Here's the drawing with two shaded views (mm, measured from the low corner). I have some questions. A direction names the side the tool comes from. Coordinates: 2 decimals unless noted, no trailing zeros. Write each loop counter-clockwise with the first axis right and the second up, starting at its lowest first coordinate (ties: lowest second). Pieces come first, ordered by that corner, then holes.
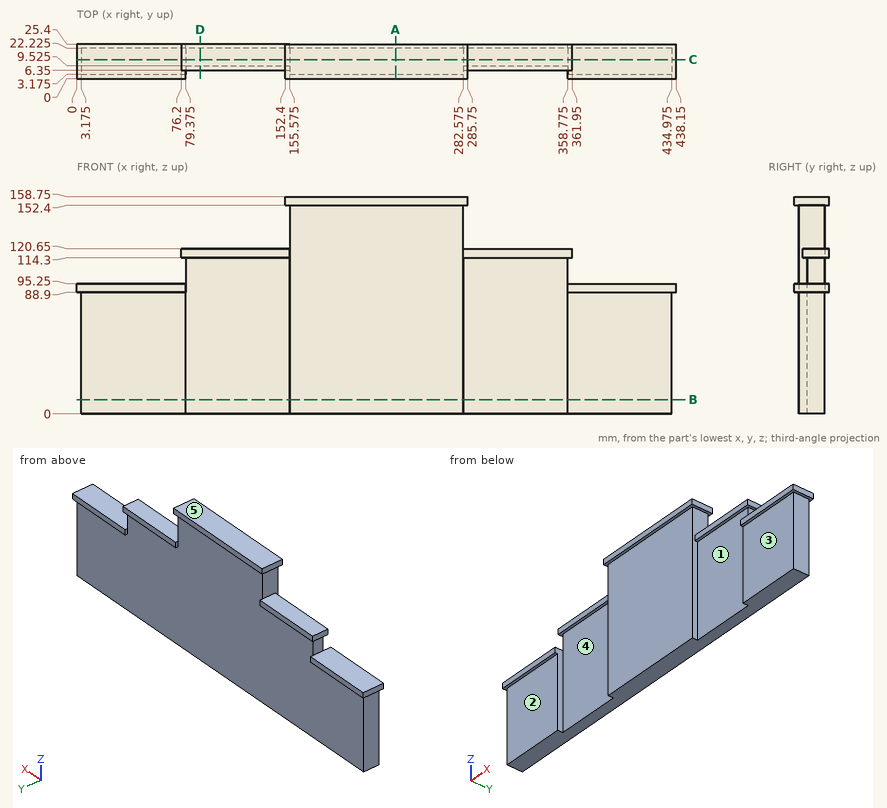
1. Please list where these lines run through material, in increasing order: line 1 along X through (y, z) = (7.25, 52.5) (3 decimals); line 2 along Z through (x, y) = (134, 18.5); line 3 along Y through (x, z) = (137, 7.5) (3 decimals).
Verdict:
line 1: x = 3.175 to 79.375, 155.575 to 282.575, 358.775 to 434.975
line 2: z = 0 to 120.65
line 3: y = 9.525 to 22.225
2. I want a section at B-B on z = 10.5. Please give me the cut outline in (x, y) (3 decimals), plus the area to 3 significant figures.
Verdict:
outline: (3.175, 3.175) - (79.375, 3.175) - (79.375, 9.525) - (155.575, 9.525) - (155.575, 3.175) - (282.575, 3.175) - (282.575, 9.525) - (358.775, 9.525) - (358.775, 3.175) - (434.975, 3.175) - (434.975, 22.225) - (3.175, 22.225) - close
area: 7,260 mm2
3. I want a section at D-D on x = 90. Please give me the cut outline in (y, z) (3 decimals), plus the area to 3 significant figures.
Verdict:
outline: (6.35, 114.3) - (9.525, 114.3) - (9.525, 0) - (22.225, 0) - (22.225, 114.3) - (25.4, 114.3) - (25.4, 120.65) - (6.35, 120.65) - close
area: 1,570 mm2
4. On a 3-axis mill with a long thin cutter (end or side, diameter ignored), from which of +Z, -Z, +X, -X, +Y, -Y can I reach the whole of each face in a straight line? I mean the marked faces 3, 4 and 5. Say none if no direction works.
Verdict:
face 3: -Z, +X, -X, -Y
face 4: -Z, -Y
face 5: +Z, +X, -X, +Y, -Y
5. I want a section at A-A on x = 233. Please give me the cut outline in (y, z) (3 decimals), plus the area to 3 significant figures.
Verdict:
outline: (0, 152.4) - (3.175, 152.4) - (3.175, 0) - (22.225, 0) - (22.225, 152.4) - (25.4, 152.4) - (25.4, 158.75) - (0, 158.75) - close
area: 3,060 mm2
6. If we mould it in two halves opening along X, with no side actions, what happens to the marked faces 1 and 2? For each: pulls with the +X half, pulls with the -X half, needs draft (parallel to the pull), parting line crosses it, or undercut.
Verdict:
face 1: undercut
face 2: needs draft
7. I want a section at C-C on y = 14. Please give me the cut outline in (x, z) (3 decimals).
Verdict:
outline: (0, 88.9) - (3.175, 88.9) - (3.175, 0) - (434.975, 0) - (434.975, 88.9) - (438.15, 88.9) - (438.15, 95.25) - (358.775, 95.25) - (358.775, 114.3) - (361.95, 114.3) - (361.95, 120.65) - (282.575, 120.65) - (282.575, 152.4) - (285.75, 152.4) - (285.75, 158.75) - (152.4, 158.75) - (152.4, 152.4) - (155.575, 152.4) - (155.575, 120.65) - (76.2, 120.65) - (76.2, 114.3) - (79.375, 114.3) - (79.375, 95.25) - (0, 95.25) - close
8. For pin 1 (3 mm diameter, centred on y = 6.5, z = 33.5, fed in from -X) (3 decimals); pin 2 (7 mm diameter, centred on x = 321, z = 118.5, fed in from -Y); pin 3 (6 mm diameter, centred on y = 5.5, z = 18.5, fed in from +X) (3 decimals), each with a flat end and sliding along its axis, tell me the tip position at first contact or that it passes through.
Verdict:
pin 1: stops at x = 3.175
pin 2: stops at y = 6.35
pin 3: stops at x = 434.975
